Geometry check sheet. Reference: the model listing, model coordinates, mm. Face numbers are marked on the shaded views. A direction names the side the tool comes from. Round coordinates to 2 decimals unless told otherwise and drop trailing zeros. Loops run counter-clockwise (first coordinate to the right, second up) from the corner with the lowest first, then second, coordinate; pieces in that order, holes last. Notation, with made-up numbers: (84.5, -30) - (93.5, -30) arc R24 cw to (93.5, 7) - close; hole circle Ø4 at (10.5, 26.25). An arc over 180 degrees is marked (long way). Write item = value, one per line.
```python
from build123d import *

# Parameters (mm, degrees)
SKETCH2_W           = 76.2
SKETCH2_H           = 6.35
BOSS_EXTRUDE1_DEPTH = 3.175
SKETCH3_R           = 1.6
BOSS_EXTRUDE2_DEPTH = 3.175
FILLET1_START       = -4
FILLET1_DEPTH       = 8
FILLET1_START_2     = -3.175
FILLET1_2_DEPTH     = 6.35
SKETCH6_R           = 4.1275
SKETCH6_R_2         = 1.725
BOSS_EXTRUDE4_DEPTH = 3.175
CHAMFER2_SIZE       = 0.254


with BuildPart() as part:
    # Sketch2 → Boss-Extrude1 (new body)
    with BuildSketch(Plane(origin=(0, 0, 0), x_dir=(1, 0, 0), z_dir=(0, 1, 0))):
        with Locations((38.1, 0)):
            Rectangle(SKETCH2_W, SKETCH2_H)
    extrude(amount=BOSS_EXTRUDE1_DEPTH)

    # Sketch3 → Boss-Extrude2 (add)
    with BuildSketch(Plane(origin=(0, 3.175, 0), x_dir=(1, 0, 0), z_dir=(0, 1, 0))):
        with BuildLine():
            Line((6.35, 3.175), (-12.7, 3.175))
            ThreePointArc((-12.7, 3.175), (-15.875, 0), (-12.7, -3.175))
            Line((-12.7, -3.175), (6.35, -3.175))
            Line((6.35, -3.175), (6.35, 3.175))
        make_face()
        with Locations(Location((-12.7, 0, 0), (0, 0, 270))):
            Circle(SKETCH3_R, mode=Mode.SUBTRACT)
        with Locations(Location((-6.35, 0, 0), (0, 0, 270))):
            Circle(SKETCH3_R, mode=Mode.SUBTRACT)
    extrude(amount=BOSS_EXTRUDE2_DEPTH)

    # Fillet1: read off the stored shape, not the designer's step
    # Fillet1 outline → Fillet1 (cut)
    with BuildSketch(Plane.XY.offset(FILLET1_START)):
        with BuildLine():
            ThreePointArc((4.7625, 6.35), (5.885032015, 5.885032015), (6.35, 4.7625))
            Line((6.35, 4.7625), (6.35, 6.35))
            Line((6.35, 6.35), (4.7625, 6.35))
        make_face()
    extrude(amount=FILLET1_DEPTH, mode=Mode.SUBTRACT)

    # Fillet1 2 outline → Fillet1 2 (add)
    with BuildSketch(Plane.XY.offset(FILLET1_START_2)):
        with BuildLine():
            ThreePointArc((7.9375, 3.175), (6.814967985, 3.639967985), (6.35, 4.7625))
            Line((6.35, 4.7625), (6.35, 3.175))
            Line((6.35, 3.175), (7.9375, 3.175))
        make_face()
    extrude(amount=FILLET1_2_DEPTH)

    # Sketch6 → Boss-Extrude4 (add)
    with BuildSketch(Plane.XY.offset(3.175)):
        with BuildLine():
            Line((76.2, 3.175), (60.96, 3.175))
            Line((60.96, 3.175), (60.96, 13.335))
            ThreePointArc((60.96, 13.335), (68.58, 20.955), (76.2, 13.335))
            Line((76.2, 13.335), (76.2, 3.175))
        make_face()
        with Locations((68.58, 10.033)):
            Circle(SKETCH6_R, mode=Mode.SUBTRACT)
        with Locations((68.58, 17.653)):
            Circle(SKETCH6_R_2, mode=Mode.SUBTRACT)
    extrude(amount=-BOSS_EXTRUDE4_DEPTH)

    # Chamfer2
    chamfer2_edges = [part.edges().sort_by_distance(p)[0] for p in [
        (66.855, 17.653, 0),
    ]]
    chamfer(chamfer2_edges, length=CHAMFER2_SIZE)


solid = part.part
```
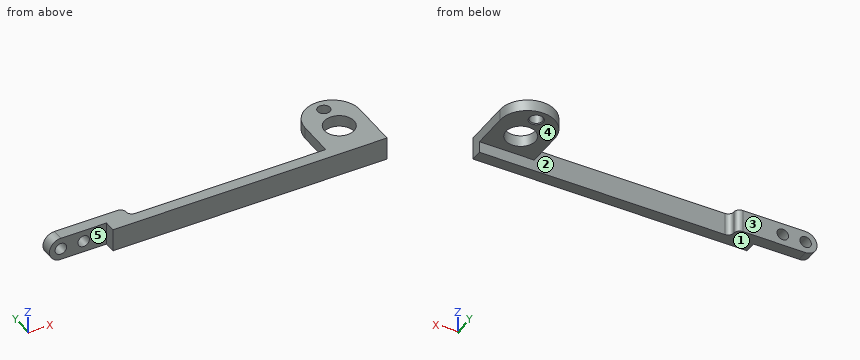
(1) Gauge pin test, flat ends, axial feed: pin 1 (1.5 mm diameter, centred on y = 11.5, z = -2, fed in from +X); pin 2 (1 mm diameter, centred on y = 5.5, z = 2, fed in from -X); pin 3 (2 mm diameter, centred on y = 18, z = 1.5, fed in from -X); pin 4 (1 mm diameter, centred on y = 1.5, z = -1, fed in from -X). Record the tip position at first contact, or that the pin passes through.
Answers follow:
pin_1 = through
pin_2 = -15.5
pin_3 = 61.9
pin_4 = 0
(2) Section check C-C (y = 11). Enter the section's corners in (x, z) (3 decimals), then the cut area to 3 significant figures.
Answers follow:
outline = (60.96, 0) - (64.567, 0) - (64.567, 3.175) - (60.96, 3.175) - close; (72.593, 0) - (76.2, 0) - (76.2, 3.175) - (72.593, 3.175) - close
area = 22.9 mm²
(3) Scan lines: L1, parallel to Y at x = 68.58, z = 2.5 (1 decimal); L2, parallel to X at y = 4, z = -0.5; L3, parallel to Y at x = 3.5, z = -2.5. Record each from-to range of solid material in increasing order. Write a range as [from, to].
Answers follow:
L1 = [0, 5.9], [14.2, 15.9], [19.4, 21]
L2 = [-15.84, -14.22], [-11.18, -7.87], [-4.83, 6.55]
L3 = [0, 6.35]
(4) Section check B-B (x = 68.58). State how many separate pieces and enclosed holes the cut face has, then the cut area to 3 significant figures.
Answers follow:
separate_pieces = 3
enclosed_holes = 0
area = 39.4 mm²
(5) Section check A-A (x = -6.35). Enter the section's corners in (y, z) (3 decimals), then the cut area to 3 significant figures.
Answers follow:
outline = (3.175, -3.175) - (6.35, -3.175) - (6.35, -1.6) - (3.175, -1.6) - close; (3.175, 1.6) - (6.35, 1.6) - (6.35, 3.175) - (3.175, 3.175) - close
area = 10.0 mm²
(6) Mould release check, pull along X, two halves, no side actions. Record for the marked faces 1 and 2: pulls with the +X half, pulls with the -X half, needs draft (parallel to the pull), parting line crosses it, or undercut.
Answers follow:
face_1 = needs draft
face_2 = undercut
(7) Section check D-D (y = 1.75). Enter the section's corners in (x, z) (3 decimals).
Answers follow:
outline = (0, -3.175) - (76.2, -3.175) - (76.2, 3.175) - (0, 3.175) - close
(8) Set-up check for the marked faces 3, 4 and 5: record each of +Z, -Z, +X, -X, +Y, -Y from which the full face is reachable in a straight line by a thin tool's end or side.
Answers follow:
face_3 = +Z, -Z, -X, +Y
face_4 = -Z, +X, +Y
face_5 = +Z, -Z, -X, -Y
